```python
from build123d import *

# Parameters (mm, degrees)
F0_W     = 25
F0_H     = 25
F0_W_2   = 12
F0_H_2   = 4
F1_DEPTH = 40
F2_W     = 1.5
F2_H     = 6
F3_DEPTH = 15
F4_R     = 1.75
F5_DEPTH = 25
F6_W     = 12
F6_H     = 4
F7_DEPTH = 25
F8_R     = 5


with BuildPart() as f1:
    # F0 (on Top) → F1 (new body)
    with BuildSketch(Plane.XY):
        Rectangle(F0_W, F0_H)
        with Locations((0, 5.5)):
            Rectangle(F0_W_2, F0_H_2, mode=Mode.SUBTRACT)
    extrude(amount=F1_DEPTH)

    # F2 (on face) → F3 (join)
    with BuildSketch(Plane(origin=(0, 0, 0), x_dir=(1, 0, 0), z_dir=(0, 0, -1))):
        with Locations((-7.75, 0)):
            Rectangle(F2_W, F2_H)
        with Locations((7.75, 0)):
            Rectangle(F2_W, F2_H)
    extrude(amount=F3_DEPTH)

    # F4 (on face) → F5 (cut)
    with BuildSketch(Plane(origin=(-8.5, 0, 0), x_dir=(0, -1, 0), z_dir=(-1, 0, 0))):
        with Locations((0, -11.713912)):
            Circle(F4_R)
    extrude(amount=-F5_DEPTH, mode=Mode.SUBTRACT)

    # F6 (on face) → F7 (join)
    with BuildSketch(Plane(origin=(0, 0, 0), x_dir=(1, 0, 0), z_dir=(0, 0, -1))):
        with Locations((0, -5.5)):
            Rectangle(F6_W, F6_H)
    extrude(amount=-F7_DEPTH)

    # F8
    f8_edges = [f1.edges().sort_by_distance(p)[0] for p in [
        (12.5, 12.5, 20),
        (-12.5, 12.5, 20),
        (12.5, -12.5, 20),
        (-12.5, -12.5, 20),
    ]]
    fillet(f8_edges, radius=F8_R)


solid = f1.part
```
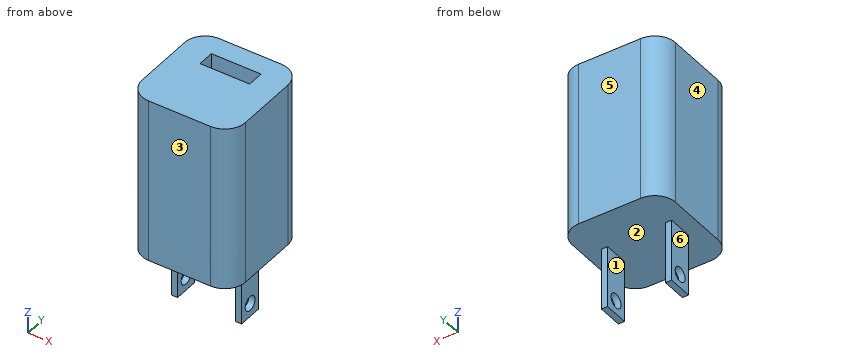
For this review, take the finished solid that the model builds, in its own axes (mm). Face numbers are marked on the shaded views. A direction names the side the tool comes from. Coordinates: 2 decimals unless noted, no trailing zeros. Loops run counter-clockwise (first coordinate to the right, second up) from the corner with the lowest first, then second, coordinate; pieces in that order, holes last.
1. Insertion check: P1, Ø4, axis at x = -4, y = 4, coming from the -Z side; P2, Ø5, axis at y = 0.5, z = -11, coming from the -X side; P3, Ø4.5, axis at y = 0, z = -11.71, coming from the +X side; P4, Ø5, axis at y = -9.5, z = 31, coming from the -X side. Each pin has a flat end and moves straight along its axis. Give the tip position at first contact, or say it passes through.
2. Add section B-B, the plane y = 0. Give the boundary of the cut face in (x, z).
3. For line 1 (Z direction, x = 7.7, y = 0); line 2 (Z direction, x = 4.25, y = 11.25); line 3 (X direction, y = -11, z = 16), list the stretches that pass through material, from the lowest coordinate up.
4. Add section D-D, the plane x = -2.5. Give the boundary of the cut face in (y, z), then the cut area to 3 significant figures.
5. Mouldability with a two-part tool opening along X and no side actions: class the marked faces 1, 2, 3 and 4 as +X half, -X half, draft (parallel to the pull), parting line (faces both ways), or undercut.
6. Add section A-A, the plane z = 29.5. Give the boundary of the cut face in (x, y).
7. Add section C-C, the plane y = 6.5. Give the boundary of the cut face in (x, z), then the cut area to 3 significant figures.
8. For the marked faces 5 and 6, list the 3-axis set-ups (+Z, -Z, +X, -X, +Y, -Y) from which the entire face can be reached by the end or side of a thin tool; tool diameter is ignored.
Result:
1. P1: stops at z = 0
1. P2: stops at x = -8.5
1. P3: stops at x = 8.5
1. P4: stops at x = -12.5
2. outline: (-12.5, 0) - (-8.5, 0) - (-8.5, -9.96) - (-7, -9.96) - (-7, 0) - (7, 0) - (7, -9.96) - (8.5, -9.96) - (8.5, 0) - (12.5, 0) - (12.5, 40) - (-12.5, 40) - close; (-8.5, -15) - (-7, -15) - (-7, -13.46) - (-8.5, -13.46) - close; (7, -15) - (8.5, -15) - (8.5, -13.46) - (7, -13.46) - close
3. line 1: z = -15 to -13.46, -9.96 to 40
3. line 2: z = 0 to 40
3. line 3: x = -11.07 to 11.07
4. outline: (-12.5, 0) - (12.5, 0) - (12.5, 40) - (7.5, 40) - (7.5, 25) - (3.5, 25) - (3.5, 40) - (-12.5, 40) - close
4. area: 940 mm2
5. face 1: undercut
5. face 2: undercut
5. face 3: draft
5. face 4: -X half
6. outline: (-12.5, -7.5) arc R5 ccw to (-7.5, -12.5) - (7.5, -12.5) arc R5 ccw to (12.5, -7.5) - (12.5, 7.5) arc R5 ccw to (7.5, 12.5) - (-7.5, 12.5) arc R5 ccw to (-12.5, 7.5) - close; hole (-6, 3.5) - (6, 3.5) - (6, 7.5) - (-6, 7.5) - close
7. outline: (-12.5, 0) - (12.5, 0) - (12.5, 40) - (6, 40) - (6, 25) - (-6, 25) - (-6, 40) - (-12.5, 40) - close
7. area: 820 mm2
8. face 5: +Z, -Z, +X, -X, +Y
8. face 6: -Z, -X, +Y, -Y
